Autodesk Inventor part; units mm, degrees
ref_plane "YZ Plane" through (0, 0, 0) normal (1, 0, 0) x (0, 1, 0)
ref_plane "XZ Plane" through (0, 0, 0) normal (0, 1, 0) x (-1, 0, 0)
ref_plane "XY Plane" through (0, 0, 0) normal (0, 0, 1) x (1, 0, 0)
sketch "スケッチ1" plane through (0, 0, 0) normal (0, 0, 1) x (1, 0, 0)
  line L0 (3.0278, 0.9571) -> (2.3427, -2.1436)
  line L1 (2.3427, -2.1436) -> (-0.6851, -3.1007)
  line L2 (-0.6851, -3.1007) -> (-3.0278, -0.9571)
  line L3 (-3.0278, -0.9571) -> (-2.3427, 2.1436)
  line L4 (-2.3427, 2.1436) -> (0.6851, 3.1007)
  line L5 (0.6851, 3.1007) -> (3.0278, 0.9571)
  circle A0 centre (0, 0) radius 2.75
  dimension "d0" = 6.3509
  dimension "d1" = 5.5
extrude "押し出し1" add sketch "スケッチ1" along normal blind 1 contours A0
extrude "押し出し2" add sketch "スケッチ1" against normal blind 3
hole "穴1" at (0, 0, 0) direction (0, 0, -1) diameter 2.5 end through all
hole "穴2" at (0, 0, 0) direction (0, 0, 1) diameter 2.5 end through all
properties part number "ナイロンナットm3" material "ステンレス鋼"
Can you work these out from the model? Positions are in its coordinate system, mm. A direction names the side the tool comes from. Coordinates: 2 decimals unless noted, no trailing zeros. Write each loop counter-clockwise with the first axis right and the second up, starting at its lowest first coordinate (ties: lowest second). Pieces come first, ordered by that corner, then holes. Notation, with made-up numbers: M -22,15.25 L 29,15.25 A15 ccw 29,44.25 Z; hole C -21.5,15.5 d3. An arc over 180 degrees is marked long. Write item = value, one per line. Start each with the question number.
Q1. If I drill on L1, parallel to X at y = 0, z = 0.1; L2, parallel to Z at x = -1.25, y = -2.5, over which ranges is the centre line in solid material (lowest first)? Write a range as [from, to].
Q2. If we section it at A-A, the plane z = -1.4: Write out the boundary of the cut face in (x, y), then the cut area to 3 significant figures.
Q3. I'm going to push flat-ended pins straight in: pin 1 (1 mm diameter, centred on x = -2, z = -2.5, fed in from +Y); pin 2 (1 mm diameter, centred on x = -2.5, z = -1, fed in from +Y). Where does each tip first touch, or does it pass through?
Q4. On a 3-axis mill with a long thin cutter (end or side, diameter ignored), from which of +Z, -Z, +X, -X, +Y, -Y can I reach the whole of each face in a straight line? I mean faces 1 (the face through (2.2, -1.9, 0)), 2 (the face through (1, -1, 1)), 3 (the face through (-2.11, 1.99, 0)). Say none if no direction works.
Q5. If we section it at C-C, the plane x = 0: Write out the boundary of the cut face in (y, z).
Check sheet entries:
q1.L1 = [-2.75, -1.25], [1.25, 2.75]
q1.L2 = [-3, 0]
q2.outline = M -3.03,-0.96 L -0.69,-3.1 L 2.34,-2.14 L 3.03,0.96 L 0.69,3.1 L -2.34,2.14 Z; hole C 0,0 d2.5
q2.area = 21.3 mm²
q3.pin_1 = 2.41
q3.pin_2 = 2.25
q4.face_1 = +Z, +X, -Y
q4.face_2 = +Z, +X, -X, +Y, -Y
q4.face_3 = +Z, -X, +Y
q5.outline = M -2.88,-3 L -1.25,-3 L -1.25,1 L -2.75,1 L -2.75,0 L -2.88,0 Z; M 1.25,-3 L 2.88,-3 L 2.88,0 L 2.75,0 L 2.75,1 L 1.25,1 Z
